The figure shows three views and two pictorial views of one solid part (mm, origin at its lowest corner). Answer the questions. A direction names the side the tool comes from. Give positions to 0.01 mm unless a question says otherwise; leave off trailing zeros. Loops run counter-clockwise (first coordinate to the right, second up) from the corner with the lowest first, then second, coordinate; pieces in that order, holes last. Notation, with made-up numbers: (45, -1.5) - (95, -1.5) arc R27 cw to (95, 33.5) - close; hole circle Ø10 at (-14, 13.5). An arc over 180 degrees is marked (long way). Use CSV: the item, a comma, the result in double quotes.
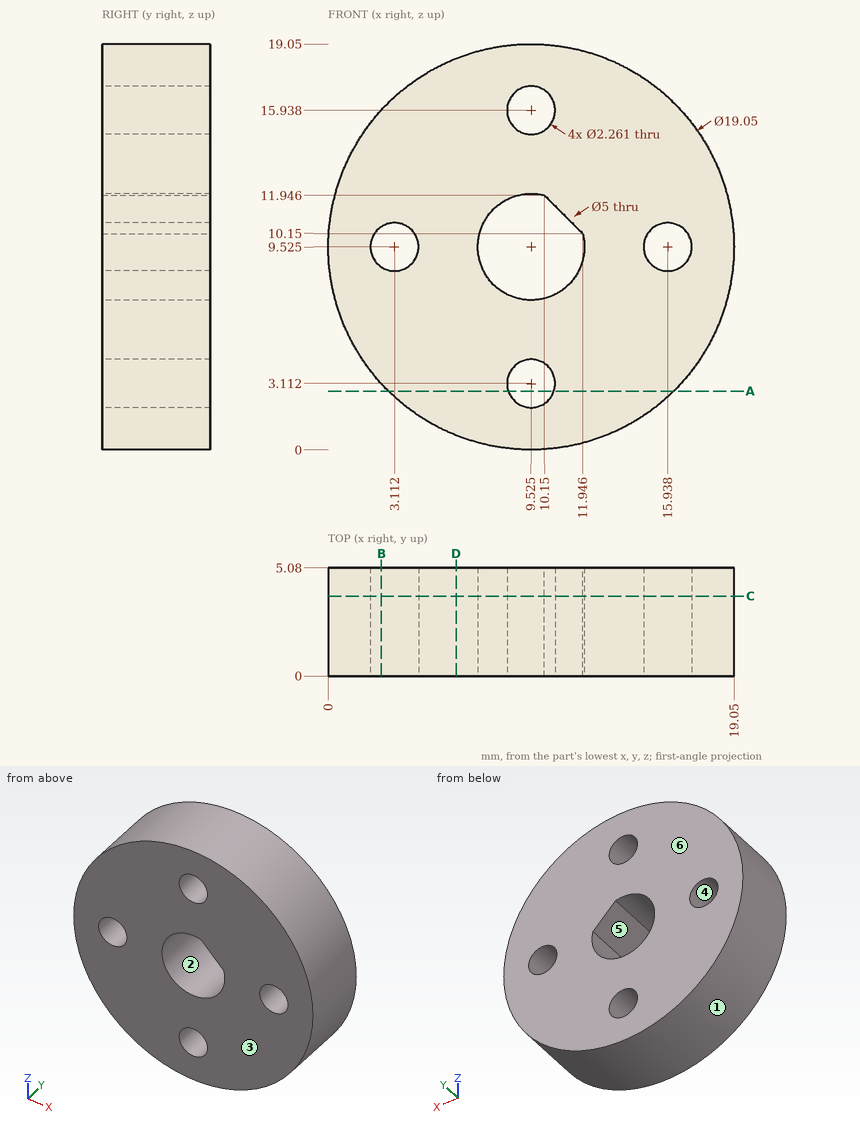
Item 1: The mould has two halves that part along Z. Classify the marked faces 1, 2, 3 and 4: pulls with the +Z half, pulls with the -Z half, needs draft (parallel to the pull), parting line crosses it, or undercut.
Determined:
face 1,"parting line crosses it"
face 2,"undercut"
face 3,"needs draft"
face 4,"undercut"
Item 2: For the marked faces 5 and 6, determine the directions among +Z, -Z, +X, -X, +Y, -Y from which every point of the face is accessible in a straight line to the end or side of a thin tool.
Determined:
face 5,"+Y, -Y"
face 6,"+Z, -Z, +X, -X, +Y"
Item 3: A cutting plane is placed at D-D on x = 6. Determine the outline of the cut face in (y, z), and give its area (3 significant figures).
Determined:
outline,"(0, 0.68) - (5.08, 0.68) - (5.08, 18.37) - (0, 18.37) - close"
area,"89.9 mm²"
Item 4: Given P1, Ø1.4, axis at x = 9.52, z = 15.94, coming from the +Y side; P2, Ø2, axis at x = 8, y = 4, coming from the +Z side; P3, Ø3, axis at y = 1.5, z = 3, coming from the -X side; P4, Ø3, axis at x = 5.5, y = 1, coming from the +Z side, each flat-ended and moving along its own axis, determine where each tip first touches the part or whether it passes through.
Determined:
P1,"passes through"
P2,"stops at z = 19.04"
P3,"stops at x = 1.43"
P4,"stops at z = 18.71"
Item 5: A cutting plane is placed at C-C on y = 3.75. State how many separate pieces and enclosed holes the cut face has, and give its area (3 significant figures).
Determined:
separate pieces,"1"
enclosed holes,"5"
area,"250 mm²"
Item 6: A cutting plane is placed at B-B on x = 2.5. Determine the outline of the cut face in (y, z) (1 decimal), and give its area (3 significant figures).
Determined:
outline,"(0, 3.1) - (5.1, 3.1) - (5.1, 8.6) - (0, 8.6) - close; (0, 10.5) - (5.1, 10.5) - (5.1, 16) - (0, 16) - close"
area,"55.7 mm²"
Item 7: A cutting plane is placed at A-A on z = 2.75. Determine the outline of the cut face in (x, y) (1 decimal).
Determined:
outline,"(2.8, 0) - (8.5, 0) - (8.5, 5.1) - (2.8, 5.1) - close; (10.6, 0) - (16.2, 0) - (16.2, 5.1) - (10.6, 5.1) - close"
Item 8: Find the intervals of material crossed by line 1 (X direction, y = 1.8, z = 3.5) (1 decimal); line 2 (X direction, y = 3.4, z = 16) (1 decimal); line 3 (Z direction, x = 7.25, y = 1) (1 decimal), in increasing order.
Determined:
line 1,"x = 2.1 to 8.5, 10.6 to 16.9"
line 2,"x = 2.5 to 8.4, 10.7 to 16.5"
line 3,"z = 0.3 to 8.5, 10.6 to 18.8"
